Here's how the part is built. I have some questions about the finished solid (model axes, mm). A direction names the side the tool comes from. Round coordinates to 2 decimals unless told otherwise and drop trailing zeros. Loops run counter-clockwise (first coordinate to the right, second up) from the corner with the lowest first, then second, coordinate; pieces in that order, holes last. Notation, with made-up numbers: M 69.25,-31 L 125.25,-31 A9 ccw 125.25,-15 Z; hole C -12,31 d3. An arc over 180 degrees is marked long. Answer as a JSON object with one key per item and string values.
from build123d import *

# Parameters (mm, degrees)
BOSS_EXTRUDE1_DEPTH = 3
FILLET1_R           = 5
FILLET2_R           = 2.5


with BuildPart() as part:
    # Sketch1 → Boss-Extrude1 (new body)
    with BuildSketch(Plane.XY):
        Polygon((-5, -25), (-5, -159), (-25, -159), (-25, -169), (-16.1, -169), (-16.1, -166.5), (-18.6, -166.5), (-18.6, -164.5), (-16.1, -164.5), (-16.1, -162), (-13.9, -162), (-13.9, -164.5), (-11.4, -164.5), (-11.4, -166.5), (-13.9, -166.5), (-13.9, -169), (-5, -169), (-5, -175), (-1.5, -175), (-1.5, -159), (1.5, -159), (1.5, -175), (5, -175), (5, -169), (13.9, -169), (13.9, -166.5), (11.4, -166.5), (11.4, -164.5), (13.9, -164.5), (13.9, -162), (16.1, -162), (16.1, -164.5), (18.6, -164.5), (18.6, -166.5), (16.1, -166.5), (16.1, -169), (25, -169), (25, -159), (5, -159), (5, -25), (5, -16.339741924), (28.8675, 25), (0, 25), (-28.8675, 25), (-5, -16.339741924), align=None)
    extrude(amount=BOSS_EXTRUDE1_DEPTH)

    # Fillet1
    fillet1_edges = [part.edges().sort_by_distance(p)[0] for p in [
        (-5, -16.339741924, 1.5),
        (5, -16.339741924, 1.5),
        (5, -159, 1.5),
        (25, -159, 1.5),
        (-25, -159, 1.5),
        (-5, -159, 1.5),
    ]]
    fillet(fillet1_edges, radius=FILLET1_R)

    # Fillet2
    fillet2_edges = [part.edges().sort_by_distance(p)[0] for p in [
        (-28.8675, 25, 1.5),
        (28.8675, 25, 1.5),
    ]]
    fillet(fillet2_edges, radius=FILLET2_R)


solid = part.part
Item 1: I want a section at B-B on y = -53.5. List the corners of the cut face in (x, z) for me.
Solution:
{"outline": "M -5,0 L 5,0 L 5,3 L -5,3 Z"}
Item 2: I want a section at A-A on x = -22. List the corners of the cut face in (y, z) for me, plus the area to 3 significant figures.
Solution:
{"outline": "M -169,0 L -159.42,0 L -159.42,3 L -169,3 Z; M 13.11,0 L 25,0 L 25,3 L 13.11,3 Z", "area": "64.4 mm2"}
Item 3: I want a section at C-C on x = -7.5. List the corners of the cut face in (y, z) for me, plus the area to 3 significant figures.
Solution:
{"outline": "M -169,0 L -158.33,0 L -158.33,3 L -169,3 Z; M -12.01,0 L 25,0 L 25,3 L -12.01,3 Z", "area": "143 mm2"}
Item 4: For faces 1 (the face through (-2, -52, 3)), 2 (the face through (24, -161, 2)), 3 (the face through (-23, -160, 2)), which set-ups out of +Z, -Z, +X, -X, +Y, -Y let a thin tool reach every point of the face, with its end or its side?
Solution:
{"face 1": "+Z, +X, -X, +Y, -Y", "face 2": "+Z, -Z, +X", "face 3": "+Z, -Z, -X"}
Item 5: We'd pull the mould along Y, two halves only. Please class faces 4 (the face through (-2, -52, 0)), 5 (the face through (16.04, 2.78, 1.48)), 6 (the face through (-7, -158, 2)): +Y half, -Y half, draft (parallel to the pull), parting line (faces both ways), or undercut.
Solution:
{"face 4": "draft", "face 5": "undercut", "face 6": "undercut"}
Item 6: For P1, Ø1, axis at y = -154.5, z = 2, coming from the -X side; P2, Ø0.8, axis at y = -163, z = 1.5, coming from the +X side; P3, Ø1.5, axis at x = 10, z = 2, coming from the -Y side, each with a flat end and sliding along its axis, tell me the tip position at first contact or that it passes through.
Solution:
{"P1": "stops at x = -5.1", "P2": "stops at x = 24.96", "P3": "stops at y = -169"}
Item 7: I want a section at D-D on y = -13. List the corners of the cut face in (x, z) for me, plus the area to 3 significant figures.
Solution:
{"outline": "M -6.93,0 L 6.93,0 L 6.93,3 L -6.93,3 Z", "area": "41.6 mm2"}
Item 8: If I drill on L1, parallel to X at y = -167, z = 2.05; L2, parallel to Y at x = 11.5, z = 2.3; L3, parallel to Y at x = 17, z = 1.85, over which ranges is the centre line in solid material (lowest first)? Write a range as from..to.
Solution:
{"L1": "x = -25..-16.1, -13.9..-1.5, 1.5..13.9, 16.1..25", "L2": "y = -169..-166.5, -164.5..-159, -5.08..25", "L3": "y = -169..-166.5, -164.5..-159, 4.44..25"}
